from build123d import *

# Parameters (mm, degrees)
F0_R     = 5.925
F1_DEPTH = 24.6
F2_R     = 4.865
F3_DEPTH = 25.9
F4_R     = 5.925
F4_R_2   = 4.865
F5_DEPTH = 28.9
F7_D     = 4.26


with BuildPart() as f1:
    # F0 (on Right) → F1 (new body)
    with BuildSketch(Plane.YZ):
        Circle(F0_R)
    extrude(amount=F1_DEPTH)

    # F2 (on face) → F3 (join)
    with BuildSketch(Plane.YZ.offset(24.6)):
        Circle(F2_R)
    extrude(amount=F3_DEPTH)

    # F4 (on face) → F5 (join)
    with BuildSketch(Plane.YZ.offset(50.5)):
        Circle(F4_R)
        Circle(F4_R_2, mode=Mode.SUBTRACT)
        Circle(F4_R_2)
    extrude(amount=F5_DEPTH)

    # F7 (through all)
    with Locations(Plane.YZ.offset(79.4)):
        with Locations((0, 0)):
            Hole(F7_D / 2)


solid = f1.part
Input: part model. Units: mm. Frame: model coordinates. A direction names the side the tool comes from. Give positions to 0.01 mm unless a question says otherwise; leave off trailing zeros. Write each loop counter-clockwise with the first axis right and the second up, starting at its lowest first coordinate (ties: lowest second). Pieces come first, ordered by that corner, then holes.
Q1. First-contact query: P1, Ø6, axis at x = 33, z = -4.5, coming from the +Y side. Flat tip, straight axial feed; report the tip coordinate or a pass-through.
Q2. Section A-A, the plane z = 0. Output: boundary loops of the cut face in (x, y) (3 decimals), plus the area to 3 significant figures.
Q3. Section D-D, the plane z = 3. Output: boundary loops of the cut face in (x, y).
Q4. Section C-C, the plane x = 46. Output: boundary loops of the cut face in (y, z) (3 decimals).
Q5. Set-up query: faces 1 (the face through (24.6, -1, 5)), 2 (the face through (79.4, 0, -3)). Return all of +Z, -Z, +X, -X, +Y, -Y with unobstructed straight access to the full face (end or side cutting, diameter ignored); none if empty.
Q6. Pull-direction query (Z, two-part tool) for faces 3 (the face through (37.37, -1.05, -4.75)), 4 (the face through (50.5, -1, 5)), 5 (the face through (39.14, 0.46, -2.08)); classes: pulls with the +Z half, pulls with the -Z half, needs draft (parallel to the pull), parting line crosses it, or undercut.
Q7. Material intervals for probe 1 along Z at (x, y) = (59.5, 0) (3 decimals); probe 2 along X at (y, z) = (-4.5, 2.5); probe 3 along Z at (x, y) = (43, 0) (3 decimals), sorted ascending.
Filled in:
1. P1: stops at y = 4.63
2. outline: (0, -5.925) - (24.6, -5.925) - (24.6, -4.865) - (50.5, -4.865) - (50.5, -5.925) - (79.4, -5.925) - (79.4, -2.13) - (0, -2.13) - close; (0, 2.13) - (79.4, 2.13) - (79.4, 5.925) - (50.5, 5.925) - (50.5, 4.865) - (24.6, 4.865) - (24.6, 5.925) - (0, 5.925) - close
2. area: 548 mm2
3. outline: (0, -5.11) - (24.6, -5.11) - (24.6, -3.83) - (50.5, -3.83) - (50.5, -5.11) - (79.4, -5.11) - (79.4, 5.11) - (50.5, 5.11) - (50.5, 3.83) - (24.6, 3.83) - (24.6, 5.11) - (0, 5.11) - close
4. outline: circle Ø9.73 at (0, 0); hole circle Ø4.26 at (0, 0)
5. face 1: none
5. face 2: +Z, -Z, +X, +Y, -Y
6. face 3: parting line crosses it
6. face 4: needs draft
6. face 5: undercut
7. probe 1: z = -5.925 to -2.13, 2.13 to 5.925
7. probe 2: x = 0 to 24.6, 50.5 to 79.4
7. probe 3: z = -4.865 to -2.13, 2.13 to 4.865
